Geometry: final body of the model. Coordinates: model frame, mm. Face numbers are marked on the shaded views. A direction names the side the tool comes from. Give positions to 0.01 mm unless a question says otherwise; leave off trailing zeros. Write each loop counter-clockwise with the first axis right and the second up, starting at its lowest first coordinate (ties: lowest second). Pieces come first, ordered by that corner, then holes.
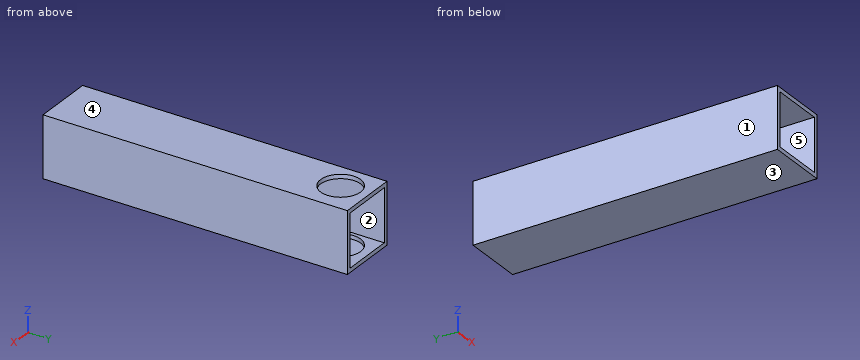
from build123d import *

# Parameters (mm, degrees)
SKETCH1_W           = 25.366424343
SKETCH1_H           = 25.503811798
BOSS_EXTRUDE1_DEPTH = 127
SKETCH2_R           = 8.338941436
CUT_EXTRUDE1_DEPTH  = 25.4
SKETCH3_W           = 21.861224343
SKETCH3_H           = 21.998611798
CUT_EXTRUDE2_DEPTH  = 127


with BuildPart() as part:
    # Sketch1 → Boss-Extrude1 (new body)
    with BuildSketch(Plane(origin=(0, 0, 0), x_dir=(1, 0, 0), z_dir=(0, 1, 0))):
        with Locations((12.683212172, -12.751905899)):
            Rectangle(SKETCH1_W, SKETCH1_H)
    extrude(amount=BOSS_EXTRUDE1_DEPTH)

    # Sketch2 → Cut-Extrude1 (cut)
    with BuildSketch(Plane.XY.offset(25.503811798)):
        with Locations((11.568608199, 115.201083313)):
            Circle(SKETCH2_R)
    extrude(amount=-CUT_EXTRUDE1_DEPTH, mode=Mode.SUBTRACT)

    # Sketch3 → Cut-Extrude2 (cut)
    with BuildSketch(Plane(origin=(0, 127, 0), x_dir=(1, 0, 0), z_dir=(0, 1, 0))):
        with Locations((12.683212172, -12.751905899)):
            Rectangle(SKETCH3_W, SKETCH3_H)
    extrude(amount=-CUT_EXTRUDE2_DEPTH, mode=Mode.SUBTRACT)


solid = part.part
Q1. Section A-A on z = 6. Output: boundary loops of the cut face in (x, y), plus the area to 3 significant figures.
Filled sheet:
outline: (0, 0) - (1.75, 0) - (1.75, 127) - (0, 127) - close; (23.61, 0) - (25.37, 0) - (25.37, 127) - (23.61, 127) - close
area: 445 mm2
Q2. Pull-direction query (Z, two-part tool) for the marked faces 3, 4 and 5; classes: released by +Z, released by -Z, zero draft, split by the parting line, or undercut.
Filled sheet:
face 3: released by -Z
face 4: released by +Z
face 5: undercut
Q3. Ray query, line 1 along Z through (x, y) = (14.75, 54.5); line 2 along X through (y, z) = (87, 7.25); line 3 along X through (y, z) = (116, 1). Return the intervals inside material, ascending.
Filled sheet:
line 1: z = 0 to 1.75, 23.75 to 25.5
line 2: x = 0 to 1.75, 23.61 to 25.37
line 3: x = 0 to 3.27, 19.87 to 25.37
Q4. Pin query (flat end, axial travel): P1, Ø10, axis at x = 11.57, y = 115.2, coming from the +Z side. Return the tip coordinate at first contact, or that it passes through.
Filled sheet:
P1: stops at z = 0.1
Q5. Section B-B on x = 11.5. Output: boundary loops of the cut face in (y, z).
Filled sheet:
outline: (0, 0) - (127, 0) - (127, 1.75) - (123.54, 1.75) - (123.54, 0.1) - (106.86, 0.1) - (106.86, 1.75) - (0, 1.75) - close; (0, 23.75) - (106.86, 23.75) - (106.86, 25.5) - (0, 25.5) - close; (123.54, 23.75) - (127, 23.75) - (127, 25.5) - (123.54, 25.5) - close
Q6. Section D-D on y = 114. Output: boundary loops of the cut face in (x, z), plus the area to 3 significant figures.
Filled sheet:
outline: (0, 0) - (25.37, 0) - (25.37, 25.5) - (19.82, 25.5) - (19.82, 23.75) - (23.61, 23.75) - (23.61, 1.75) - (19.82, 1.75) - (19.82, 0.1) - (3.32, 0.1) - (3.32, 1.75) - (1.75, 1.75) - (1.75, 23.75) - (3.32, 23.75) - (3.32, 25.5) - (0, 25.5) - close
area: 110 mm2
Q7. Section C-C on y = 66. Output: boundary loops of the cut face in (x, z).
Filled sheet:
outline: (0, 0) - (25.37, 0) - (25.37, 25.5) - (0, 25.5) - close; hole (1.75, 1.75) - (23.61, 1.75) - (23.61, 23.75) - (1.75, 23.75) - close
Q8. Access query for the marked faces 1 and 2. Directions: +Z, -Z, +X, -X, +Y, -Y. A direction counts if a zero-diameter tool reaches every point of the face in a straight line with its end or side. Return the directions, or none.
Filled sheet:
face 1: +Z, -Z, -X, +Y, -Y
face 2: +Y, -Y
